Part model, mm, in its own coordinate system. A direction names the side the tool comes from. Coordinates: 2 decimals unless noted, no trailing zeros. Order: outer loops, then holes, each group sorted by start corner. A loop starts at its lowest first (then second) coordinate and runs counter-clockwise, first axis right, second up. Notation, with made-up numbers: M 42.5,77.25 L 82.5,77.25 A17 cw 82.5,90.25 Z; hole C 48.25,21 d5. An arc over 180 degrees is marked long. Write item = value, one per line. Start each with the question number.
from build123d import *
from OCP.BRepFilletAPI import BRepFilletAPI_MakeChamfer

# Parameters (mm, degrees)
SKETCH1_R                = 22.5
BOSS_EXTRUDE1_DEPTH      = 28
SKETCH2_W                = 10.3
SKETCH2_H                = 10.3
CUT_EXTRUDE2_DEPTH       = 43.385138905
SHELL3_T                 = -2
SKETCH3_R                = 3.1
CUT_EXTRUDE3_DEPTH       = 47.576523056
CHAMFER1_SIZE            = 2
CHAMFER1_SIZE2           = 1.154700538
BOSS_EXTRUDE8_START      = 23
BOSS_EXTRUDE8_DEPTH      = 23
BOSS_EXTRUDE4_DEPTH      = 20
BOSS_EXTRUDE6_DEPTH      = 26
CUT_EXTRUDE5_DEPTH       = 12
CUT_EXTRUDE9_DEPTH       = 2
BOSS_EXTRUDE10_START     = 7
BOSS_EXTRUDE10_DEPTH     = 7
SKETCH21_OUTSIDE_W       = 61.262
SKETCH21_OUTSIDE_H       = 63.966
SKETCH21_OUTSIDE_R       = 18
CUT_EXTRUDE11_DEPTH      = 4.8
CUT_EXTRUDE12_DEPTH      = 47.730672242
CUT_EXTRUDE12_DEPTH_BACK = 47.730672242
SKETCH22_R               = 1.6
CUT_EXTRUDE13_START      = -8.5
SKETCH24_R               = 3.25
CUT_EXTRUDE13_DEPTH      = 39.230672302
CUT_EXTRUDE14_START      = -8.5
CUT_EXTRUDE14_DEPTH      = 39.230672304
FILLET1_R                = 1.5
SKETCH26_R               = 43.919943133
SKETCH26_R_2             = 22.5
CUT_EXTRUDE15_DEPTH      = 44.880328541


with BuildPart() as part:
    # Sketch1 → Boss-Extrude1 (new body)
    with BuildSketch(Plane(origin=(0, 0, 0), x_dir=(1, 0, 0), z_dir=(0, 1, 0))):
        with Locations(Location((0, 0, 0), (0, 0, 270))):
            Circle(SKETCH1_R)
    extrude(amount=BOSS_EXTRUDE1_DEPTH)

    # Sketch2 → Cut-Extrude2 (cut, through all)
    with BuildSketch(Plane.XZ):
        Rectangle(SKETCH2_W, SKETCH2_H)
    extrude(amount=-CUT_EXTRUDE2_DEPTH, mode=Mode.SUBTRACT)

    # Shell3
    shell3_openings = [part.faces().sort_by_distance(p)[0] for p in [
        (0, 0, -21.863603897),
    ]]
    offset(amount=SHELL3_T, openings=shell3_openings, kind=Kind.INTERSECTION)

    # Sketch3 → Cut-Extrude3 (cut, through all)
    with BuildSketch(Plane.XY.offset(7.15)):
        with Locations(Location((0, 15, 0), (0, 0, 270.000000016))):
            Circle(SKETCH3_R)
    extrude(amount=CUT_EXTRUDE3_DEPTH, mode=Mode.SUBTRACT)

    # Chamfer1: one chamfer whose edges measure the first distance from different faces: ONE call of the kernel's chamfer builder (chamfer() names one face for all edges)
    chamfer1_edges_1 = [part.edges().sort_by_distance(p)[0] for p in [
        (5.15, 28, 0),
    ]]
    chamfer1_side_1 = [part.faces().sort_by_distance(p)[0] for p in [
        (5.15, 14, 0),
    ]]
    chamfer1_edges_2 = [part.edges().sort_by_distance(p)[0] for p in [
        (0, 28, -5.15),
    ]]
    chamfer1_side_2 = [part.faces().sort_by_distance(p)[0] for p in [
        (0, 14, -5.15),
    ]]
    chamfer1_edges_3 = [part.edges().sort_by_distance(p)[0] for p in [
        (-5.15, 28, 0),
    ]]
    chamfer1_side_3 = [part.faces().sort_by_distance(p)[0] for p in [
        (-5.15, 14, 0),
    ]]
    chamfer1_edges_4 = [part.edges().sort_by_distance(p)[0] for p in [
        (0, 28, 5.15),
    ]]
    chamfer1_side_4 = [part.faces().sort_by_distance(p)[0] for p in [
        (0, 14, 5.15),
    ]]
    chamfer1 = BRepFilletAPI_MakeChamfer(part.part.solid().wrapped)
    for e in chamfer1_edges_1:
        chamfer1.Add(CHAMFER1_SIZE, CHAMFER1_SIZE2, e.wrapped, chamfer1_side_1[0].wrapped)  # the first distance lies on this face
    for e in chamfer1_edges_2:
        chamfer1.Add(CHAMFER1_SIZE, CHAMFER1_SIZE2, e.wrapped, chamfer1_side_2[0].wrapped)  # the first distance lies on this face
    for e in chamfer1_edges_3:
        chamfer1.Add(CHAMFER1_SIZE, CHAMFER1_SIZE2, e.wrapped, chamfer1_side_3[0].wrapped)  # the first distance lies on this face
    for e in chamfer1_edges_4:
        chamfer1.Add(CHAMFER1_SIZE, CHAMFER1_SIZE2, e.wrapped, chamfer1_side_4[0].wrapped)  # the first distance lies on this face
    add(Compound.cast(chamfer1.Shape()), mode=Mode.REPLACE)

    # Sketch18 → Boss-Extrude8 (add)
    with BuildSketch(Plane.XZ.offset(-26).offset(BOSS_EXTRUDE8_START)):
        with BuildLine():
            Line((-15.72889581, -7.671495069), (-18.425277949, -8.986608509))
            ThreePointArc((-18.425277949, -8.986608509), (-20.471905462, 1.072887103), (-17.384985971, 10.863344917))
            Line((-17.384985971, 10.863344917), (-14.840841683, 9.273587124))
            ThreePointArc((-14.840841683, 9.273587124), (-17.476016858, 0.915879234), (-15.72889581, -7.671495069))
        make_face()
    extrude(amount=-BOSS_EXTRUDE8_DEPTH)

    # Sketch9 → Boss-Extrude4 (add)
    with BuildSketch(Plane.XZ):
        Polygon((2.057061598, -22.405769292), (-16.596699733, -15.192088664), (-17.678751827, -17.990152864), (0.975009504, -25.203833492), align=None)
    extrude(amount=-BOSS_EXTRUDE4_DEPTH)

    # Sketch11 → Boss-Extrude6 (add)
    with BuildSketch(Plane.XZ):
        with BuildLine():
            Line((2.057061598, -22.405769292), (7.15, -7.15))
            Line((7.15, -7.15), (-7.15, -7.15))
            Line((-7.15, -7.15), (-16.596699733, -15.192088664))
            ThreePointArc((-16.596699733, -15.192088664), (-8.115390707, -20.985481497), (2.057061598, -22.405769292))
        make_face()
    extrude(amount=-BOSS_EXTRUDE6_DEPTH)

    # Sketch12 → Cut-Extrude5 (cut)
    with BuildSketch(Plane.XZ):
        with BuildLine():
            Line((3.835926277, -17.077224747), (2.755377072, -20.3139828))
            ThreePointArc((2.755377072, -20.3139828), (-6.94485615, -19.287793369), (-15.072724539, -13.894710323))
            Line((-15.072724539, -13.894710323), (-12.788386178, -11.950025708))
            ThreePointArc((-12.788386178, -11.950025708), (-5.15835992, -16.725347781), (3.835926277, -17.077224747))
        make_face()
    extrude(amount=-CUT_EXTRUDE5_DEPTH, mode=Mode.SUBTRACT)

    # Sketch17 → Cut-Extrude9 (cut)
    with BuildSketch(Plane.XZ):
        with BuildLine():
            Line((7.15, 7.15), (7.15, -7.15))
            Line((7.15, -7.15), (3.835926277, -17.077224747))
            ThreePointArc((3.835926277, -17.077224747), (-5.15835992, -16.725347781), (-12.788386178, -11.950025708))
            Line((-12.788386178, -11.950025708), (-7.15, -7.15))
            Line((-7.15, -7.15), (-7.15, 7.15))
            Line((-7.15, 7.15), (7.15, 7.15))
        make_face()
    extrude(amount=-CUT_EXTRUDE9_DEPTH, mode=Mode.SUBTRACT)

    # Sketch20 → Boss-Extrude10 (add)
    with BuildSketch(Plane.XZ.offset(-26).offset(BOSS_EXTRUDE10_START)):
        with BuildLine():
            Line((2.755377072, -20.3139828), (7.15, -7.15))
            Line((7.15, -7.15), (7.15, 7.15))
            Line((7.15, 7.15), (-7.15, 7.15))
            Line((-7.15, 7.15), (-7.15, -7.15))
            Line((-7.15, -7.15), (-15.072724539, -13.894710323))
            ThreePointArc((-15.072724539, -13.894710323), (6.94485615, 19.287793369), (2.755377072, -20.3139828))
        make_face()
    extrude(amount=-BOSS_EXTRUDE10_DEPTH)

    # Sketch21 outside → Cut-Extrude11 (cut)
    with BuildSketch(Plane(origin=(0, 28, 0), x_dir=(1, 0, 0), z_dir=(0, 1, 0))):
        with Locations((0, 1.352)):
            Rectangle(SKETCH21_OUTSIDE_W, SKETCH21_OUTSIDE_H)
        with Locations(Location((0, 0, 0), (0, 0, 270))):
            Circle(SKETCH21_OUTSIDE_R, mode=Mode.SUBTRACT)
    extrude(amount=-CUT_EXTRUDE11_DEPTH, mode=Mode.SUBTRACT)

    # Sketch22 → Cut-Extrude12 (cut, two sides: drawn at the far end of the back side and taken through both)
    with BuildSketch(Plane.ZY.offset(-5.15).offset(-CUT_EXTRUDE12_DEPTH_BACK)):
        with Locations((0, 23)):
            Circle(SKETCH22_R)
    extrude(amount=CUT_EXTRUDE12_DEPTH + CUT_EXTRUDE12_DEPTH_BACK, mode=Mode.SUBTRACT)

    # Sketch24 → Cut-Extrude13 (cut, through all)
    with BuildSketch(Plane.ZY.offset(-5.15).offset(CUT_EXTRUDE13_START)):
        with Locations((0, 23)):
            Circle(SKETCH24_R)
    extrude(amount=-CUT_EXTRUDE13_DEPTH, mode=Mode.SUBTRACT)

    # Sketch25 → Cut-Extrude14 (cut, through all)
    with BuildSketch(Plane(origin=(-5.15, 0, 0), x_dir=(0, 0, -1), z_dir=(1, 0, 0)).offset(CUT_EXTRUDE14_START)):
        Polygon((0, 19.75), (2.814582562, 21.375), (2.814582562, 24.625), (0, 26.25), (-2.814582562, 24.625), (-2.814582562, 21.375), align=None)
    extrude(amount=-CUT_EXTRUDE14_DEPTH, mode=Mode.SUBTRACT)

    # Fillet1
    # the kernel refuses this fillet: 1.5 mm, written as the material it takes off along each edge
    with BuildSketch(Plane(origin=(0, 23.2, 0), x_dir=(0, 0, 1), z_dir=(1, 0, 0))) as fillet1_piece_1:
        with BuildLine():
            CenterArc((22.5 - FILLET1_R, FILLET1_R), FILLET1_R, 270, 90)
            Line((22.5, FILLET1_R), (22.5, 0))
            Line((22.5, 0), (22.5 - FILLET1_R, 0))
        make_face()
    revolve(axis=Axis((0, 23.2, 0), (0, -1, 0)), revolution_arc=92.366443414, mode=Mode.SUBTRACT)
    with BuildSketch(Plane(origin=(0, 23.2, 0), x_dir=(-0.9991402664664062, 0, 0.041457543649361384), z_dir=(0.041457543649361384, 0, 0.9991402664664062))) as fillet1_piece_2:
        with BuildLine():
            CenterArc((22.5 - FILLET1_R, FILLET1_R), FILLET1_R, 270, 90)
            Line((22.5, FILLET1_R), (22.5, 0))
            Line((22.5, 0), (22.5 - FILLET1_R, 0))
        make_face()
    revolve(axis=Axis((0, 23.2, 0), (0, -1, 0)), revolution_arc=183.648889302, mode=Mode.SUBTRACT)
    with BuildSketch(Plane(origin=(0, 23.2, 0), x_dir=(0.9997569746526436, 0, -0.022045217925738058), z_dir=(-0.022045217925738058, 0, -0.9997569746526436))) as fillet1_piece_3:
        with BuildLine():
            CenterArc((22.5 - FILLET1_R, FILLET1_R), FILLET1_R, 270, 90)
            Line((22.5, FILLET1_R), (22.5, 0))
            Line((22.5, 0), (22.5 - FILLET1_R, 0))
        make_face()
    revolve(axis=Axis((0, 23.2, 0), (0, -1, 0)), revolution_arc=91.263200277, mode=Mode.SUBTRACT)

    # Sketch26 → Cut-Extrude15 (cut, through all)
    with BuildSketch(Plane.XZ):
        Circle(SKETCH26_R)
        with Locations(Location((0, 0, 0), (0, 0, 352.392535773))):
            Circle(SKETCH26_R_2, mode=Mode.SUBTRACT)
    extrude(amount=-CUT_EXTRUDE15_DEPTH, mode=Mode.SUBTRACT)


solid = part.part
Item 1: Wall check: line 1 along X through (y, z) = (10, 0); line 2 along Y through (x, z) = (10, 0); line 3 along X through (y, z) = (4, -6.5). Give the ranges that are in metal, low to high. Write a range as [from, to].
Item 2: Cut at A-A, the plane y = 6.5. Write the cut outline in (x, z).
Item 3: Cut at B-B, the plane y = 15. Write the cut outline in (x, z), and give its area (3 significant figures).
Item 4: 3-axis set-ups, long thin cutter, end or side, ignore diameter. For faces 1 (the flat face through (0, 23.2, 19)), 2 (the cylindrical face through (17.033, 19.827, -0.705)), 3 (the flat face through (4.922, 10.381, -13.824)), 4 (the flat face through (-5.15, 14, 0)): which of +Z, -Z, +X, -X, +Y, -Y reach the whole face in a straight line?
Item 5: Flat gauge pins, fed straight in: pin 1 (1.5 mm diameter, centred on x = 12.5, y = 5, fed in from +Z); pin 2 (3 mm diameter, centred on x = -16.5, z = 1.5, fed in from -Y); pin 3 (5 mm diameter, centred on x = -9.5, y = 4, fed in from -Z); pin 4 (15.5 mm diameter, centred on x = -3, y = 12.5, fed in from +Z). Where does each tip first touch, or does it go through?
Item 6: Cut at C-C, the plane x = -2.5. Count the separate pieces of the cut face and the enclosed holes in it, and give its area (3 significant figures).
Item 7: Pull direction Z, two halves, no side cores. Call faces 5 (the flat face through (-18.2, 0, 9.9)), 6 (the flat face through (0.088, 27.014, -5.735)): pulls with the +Z half, pulls with the -Z half, needs draft (parallel to the pull), parting line crosses it, or undercut.
Filled sheet:
q1.line_1 = [-22.5, -17.5], [-7.15, -5.15], [5.15, 7.15], [20.5, 22.5]
q1.line_2 = [19, 21.4], [24.6, 28]
q1.line_3 = [-21.54, -16.25], [-7.15, 7.15], [19.44, 21.54]
q2.outline = C 0,0 d45; M -12.79,-11.95 A17.5 ccw 3.84,-17.08 L 7.15,-7.15 L 7.15,7.15 L -7.15,7.15 L -7.15,-7.15 Z; hole M -18.43,-8.99 A20.5 ccw long -17.38,10.86 L -14.84,9.27 A17.5 ccw -15.73,-7.67 Z; hole M -5.15,-5.15 L 5.15,-5.15 L 5.15,5.15 L -5.15,5.15 Z
q3.outline = M -18.43,-8.99 L -15.73,-7.67 A17.5 cw -14.84,9.27 L -17.38,10.86 A20.5 cw -3.1,20.26 L -3.1,22.29 A22.5 ccw long 3.1,22.29 L 3.1,20.26 A20.5 cw 2.76,-20.31 L 7.15,-7.15 L 7.15,7.15 L -7.15,7.15 L -7.15,-7.15 L -15.07,-13.89 A20.5 cw Z; hole M -5.15,-5.15 L 5.15,-5.15 L 5.15,5.15 L -5.15,5.15 Z
q3.area = 623 mm2
q4.face_1 = +Z, +Y
q4.face_2 = +X
q4.face_3 = -Y
q4.face_4 = +Y, -Y
q5.pin_1 = 19.19
q5.pin_2 = 3
q5.pin_3 = -21.38
q5.pin_4 = 22.5
q6.separate_pieces = 3
q6.enclosed_holes = 0
q6.area = 594 mm2
q7.face_5 = needs draft
q7.face_6 = undercut
